from build123d import *

# Parameters (mm, degrees)
F0_R     = 3.175
F0_R_2   = 1.5875
F1_DEPTH = 25.4


with BuildPart() as f1:
    # F0 (on Front) → F1 (new body)
    with BuildSketch(Plane.XZ):
        with BuildLine():
            ThreePointArc((0.6794904459, -9.5007324841), (6.9712901065, -6.4905114784), (9.525, 0))
            ThreePointArc((9.525, 0), (0, 9.525), (-9.525, 0))
            ThreePointArc((-9.525, 0), (-6.7351920908, -6.7351920908), (0, -9.525))
            Line((0, -9.525), (0.6794904459, -9.5007324841))
        make_face()
        Circle(F0_R, mode=Mode.SUBTRACT)
        with BuildLine():
            Line((36.5125, 0), (9.525, 0))
            ThreePointArc((9.525, 0), (6.9712901065, -6.4905114784), (0.6794904459, -9.5007324841))
            Line((0.6794904459, -9.5007324841), (44.45, -7.9375))
            ThreePointArc((44.45, -7.9375), (38.8373399243, -5.6126600757), (36.5125, 0))
        make_face()
        with BuildLine():
            ThreePointArc((-9.525, 0), (0, 9.525), (9.525, 0))
            Line((9.525, 0), (36.5125, 0))
            ThreePointArc((36.5125, 0), (38.8373399243, 5.6126600757), (44.45, 7.9375))
            Line((44.45, 7.9375), (18.9329889534, 8.8488218231))
            ThreePointArc((18.9329889534, 8.8488218231), (13.22446249, 11.5691841219), (11.3070069952, 17.5950458731))
            Line((11.3070069952, 17.5950458731), (15.7942028036, 61.9003804205))
            ThreePointArc((15.7942028036, 61.9003804205), (0, 47.625), (-15.7942028036, 61.9003804205))
            Line((-15.7942028036, 61.9003804205), (-9.525, 0))
        make_face()
        with BuildLine():
            ThreePointArc((0, -9.525), (0.3399618281, -9.5189311877), (0.6794904459, -9.5007324841))
            Line((0.6794904459, -9.5007324841), (0, -9.525))
        make_face()
        with BuildLine():
            ThreePointArc((44.45, 7.9375), (38.8373399243, 5.6126600757), (36.5125, 0))
            ThreePointArc((36.5125, 0), (38.8373399243, -5.6126600757), (44.45, -7.9375))
            ThreePointArc((44.45, -7.9375), (50.0626600757, -5.6126600757), (52.3875, 0))
            ThreePointArc((52.3875, 0), (50.0626600757, 5.6126600757), (44.45, 7.9375))
        make_face()
        with BuildLine():
            ThreePointArc((47.625, 0), (44.45, -3.175), (41.275, 0))
            ThreePointArc((41.275, 0), (44.45, 3.175), (47.625, 0))
        make_face(mode=Mode.SUBTRACT)
        with BuildLine():
            ThreePointArc((-15.7474569047, 65.5082893304), (-15.873667691, 63.7056672947), (-15.7942028036, 61.9003804205))
            ThreePointArc((-15.7942028036, 61.9003804205), (0, 47.625), (15.7942028036, 61.9003804205))
            ThreePointArc((15.7942028036, 61.9003804205), (15.8547878338, 62.6991705884), (15.875, 63.5))
            ThreePointArc((15.875, 63.5), (15.8430821396, 64.5061676396), (15.7474569047, 65.5082893304))
            ThreePointArc((15.7474569047, 65.5082893304), (0, 79.375), (-15.7474569047, 65.5082893304))
        make_face()
        with Locations((0, 63.5)):
            Circle(F0_R, mode=Mode.SUBTRACT)
        with BuildLine():
            Line((-9.525, 114.3), (-15.7474569047, 65.5082893304))
            ThreePointArc((-15.7474569047, 65.5082893304), (0, 79.375), (15.7474569047, 65.5082893304))
            Line((15.7474569047, 65.5082893304), (9.525, 114.3))
            ThreePointArc((9.525, 114.3), (0, 104.775), (-9.525, 114.3))
        make_face()
        with Locations((-3.4632231109, 100.0252)):
            Circle(F0_R_2, mode=Mode.SUBTRACT)
        with BuildLine():
            ThreePointArc((9.525, 114.3), (0, 123.825), (-9.525, 114.3))
            ThreePointArc((-9.525, 114.3), (0, 104.775), (9.525, 114.3))
        make_face()
        with Locations((0, 114.3)):
            Circle(F0_R, mode=Mode.SUBTRACT)
    extrude(amount=F1_DEPTH)


solid = f1.part
Source: CAD feature listing. Evaluate the final solid. Frame: model axes, mm. Give positions to 0.01 mm unless a question says otherwise; leave off trailing zeros. Write each loop counter-clockwise with the first axis right and the second up, starting at its lowest first coordinate (ties: lowest second). Pieces come first, ordered by that corner, then holes. Notation, with made-up numbers: M 84.5,-3.75 L 139.5,-3.75 A12 cw 139.5,2.25 Z; hole C -26,14 d3. An arc over 180 degrees is marked long. Answer as a JSON object with one key per item and string values.
Q1. Cut plane B-B, the plane z = 68. Return the cut outline in (x, y), then the cut area to 3 significant figures.
Geometry check:
{"outline": "M -15.43,-25.4 L 15.43,-25.4 L 15.43,0 L -15.43,0 Z", "area": "784 mm^2"}
Q2. Mould query, pull axis X, two halves, no side actions, for faces 1 (the face through (13.52, -12.52, 39.44)), 2 (the face through (-0.69, -12.52, 111.2)), 3 (the face through (0.209, -12.522, 123.823)). Classes: +X half, -X half, draft (parallel to the pull), parting line (faces both ways), or undercut.
Geometry check:
{"face 1": "+X half", "face 2": "undercut", "face 3": "parting line"}
Q3. Cut plane A-A, the plane y = -14. Count the separate pieces of the cut face and the enclosed holes in it, then the cut area to 3 significant figures.
Geometry check:
{"separate pieces": "1", "enclosed holes": "5", "area": "3,790 mm^2"}
Q4. Contact query for flat-ended pins moving along their axis: P1, Ø4, axis at x = 27, y = -14, coming from the -Z side; P2, Ø2, axis at y = -4.5, z = 105, coming from the -X side; P3, Ø8, axis at x = 41.5, y = -21, coming from the -Z side. Output: stop coordinate, or through.
Geometry check:
{"P1": "stops at z = -8.63", "P2": "stops at x = -10.84", "P3": "stops at z = -8.19"}
Q5. Ray query, line 1 along Z through (x, y) = (0, -9.75) (3 decimals); line 2 along X through (y, z) = (-4.75, 2.5); line 3 along X through (y, z) = (-20.25, -1). Return the intervals inside material, ascending.
Geometry check:
{"line 1": "z = -9.525 to -3.175, 3.175 to 60.325, 66.675 to 111.125, 117.475 to 123.825", "line 2": "x = -9.78 to -1.96, 1.96 to 42.49, 46.41 to 51.98", "line 3": "x = -9.47 to -3.01, 3.01 to 41.44, 47.46 to 52.32"}
Q6. Cut plane C-C, the plane z = 87. Return the cut outline in (x, y), then the cut area to 3 significant figures.
Geometry check:
{"outline": "M -13.01,-25.4 L 13.01,-25.4 L 13.01,0 L -13.01,0 Z", "area": "661 mm^2"}
